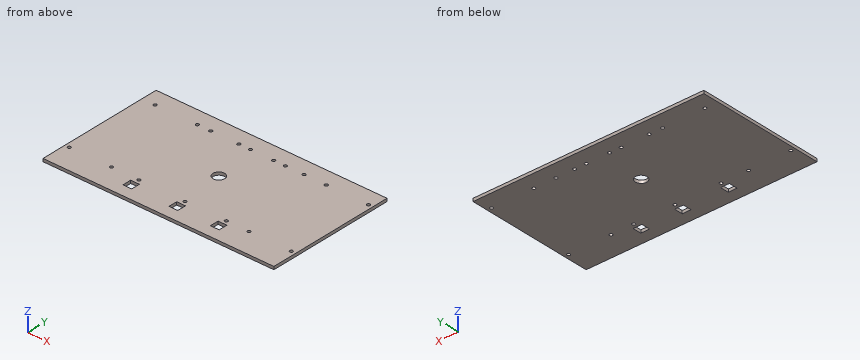
from build123d import *

# Parameters (mm, degrees)
F0_W     = 251.524948
F0_H     = 139.850774
F0_R     = 1.7272
F0_W_2   = 9.525
F0_H_2   = 9.525
F0_R_2   = 6.35
F1_DEPTH = 3.175


with BuildPart() as f1:
    # F0 (on Top) → F1 (new body)
    with BuildSketch(Plane.XY):
        with Locations((125.762474, -69.925387)):
            Rectangle(F0_W, F0_H)
        with Locations((4.7625, -112.863274)):
            Circle(F0_R, mode=Mode.SUBTRACT)
        with Locations((50.8, -112.863274)):
            Circle(F0_R, mode=Mode.SUBTRACT)
        Polygon((85.434995, -117.625774), (85.434995, -127.150774), (75.909995, -127.150774), (75.909995, -117.625774), align=None, mode=Mode.SUBTRACT)
        with Locations((80.672495, -112.863274)):
            Circle(F0_R, mode=Mode.SUBTRACT)
        with Locations((130.838715, -122.388274)):
            Rectangle(F0_W_2, F0_H_2, mode=Mode.SUBTRACT)
        with Locations((175.928693, -122.388274)):
            Rectangle(F0_W_2, F0_H_2, mode=Mode.SUBTRACT)
        with Locations((130.838715, -112.863274)):
            Circle(F0_R, mode=Mode.SUBTRACT)
        with Locations((175.928693, -112.863274)):
            Circle(F0_R, mode=Mode.SUBTRACT)
        with Locations((200.724948, -112.863274)):
            Circle(F0_R, mode=Mode.SUBTRACT)
        with Locations((246.762448, -112.863274)):
            Circle(F0_R, mode=Mode.SUBTRACT)
        with Locations((14.2875, -17.4625)):
            Circle(F0_R, mode=Mode.SUBTRACT)
        with Locations((60.325, -17.4625)):
            Circle(F0_R, mode=Mode.SUBTRACT)
        with Locations((74.93, -17.4625)):
            Circle(F0_R, mode=Mode.SUBTRACT)
        with Locations((105.464991, -17.4625)):
            Circle(F0_R, mode=Mode.SUBTRACT)
        with Locations((118.164991, -17.4625)):
            Circle(F0_R, mode=Mode.SUBTRACT)
        with Locations((125.762474, -65.162887)):
            Circle(F0_R_2, mode=Mode.SUBTRACT)
        with Locations((143.512438, -17.4625)):
            Circle(F0_R, mode=Mode.SUBTRACT)
        with Locations((156.212438, -17.4625)):
            Circle(F0_R, mode=Mode.SUBTRACT)
        with Locations((176.594948, -17.4625)):
            Circle(F0_R, mode=Mode.SUBTRACT)
        with Locations((200.724948, -17.4625)):
            Circle(F0_R, mode=Mode.SUBTRACT)
        with Locations((246.762448, -17.4625)):
            Circle(F0_R, mode=Mode.SUBTRACT)
    extrude(amount=F1_DEPTH)


solid = f1.part
Model file for the job. Use its own axes, mm. Coordinates: 2 decimals unless noted, no trailing zeros. Return JSON: item names as keys, results as strings.
1. Saw through at A-A (z = 2.05). Give the number of separate pieces and of enclosed holes in the cut face, and give its area (3 significant figures).
Ans:
{"separate pieces": "1", "enclosed holes": "21", "area": "34,600 mm^2"}
2. Drill centre lines: probe 1 along Y at (x, z) = (125.5, 0.2); probe 2 along X at (y, z) = (-65, 0.15); probe 3 along X at (y, z) = (-60, 2.05). Where is each one in solid material? Low to high.
Ans:
{"probe 1": "-139.85 to -71.51, -58.82 to 0", "probe 2": "0 to 119.41, 132.11 to 251.52", "probe 3": "0 to 122.07, 129.46 to 251.52"}
3. Flat gauge pin, fed straight in: pin 1 (2 mm diameter, centred on x = 14.29, y = -17.46, fed in from +Z). Where does the tip first touch, or does it go through?
Ans:
{"pin 1": "through"}
